Work out the finished part from the listing and answer in its coordinate system (mm). Round coordinates to 2 decimals unless told otherwise and drop trailing zeros. Loops run counter-clockwise (first coordinate to the right, second up) from the corner with the lowest first, then second, coordinate; pieces in that order, holes last. Notation, with made-up numbers: (-10, -32) -> (29, -32) arc R19 cw to (29, -18) -> close; hole circle Ø8 at (85.5, -18.75). An arc over 180 degrees is marked (long way). Write item = value, one per line. Start each with the question number.
```python
from build123d import *

# Parameters (mm, degrees)
SKETCH_W       = 190
SKETCH_H       = 82
SKETCH_R       = 1.65
PAD_DEPTH      = 0.75
PAD_DEPTH_BACK = 1.75
POCKET_DEPTH   = 5


with BuildPart() as part:
    # Sketch → Pad (new body, two sides)
    with BuildSketch(Plane.XZ) as pad_sk:
        Rectangle(SKETCH_W, SKETCH_H)
        with Locations((90, 30)):
            Circle(SKETCH_R, mode=Mode.SUBTRACT)
        with Locations((90, 10)):
            Circle(SKETCH_R, mode=Mode.SUBTRACT)
        with Locations((90, -30)):
            Circle(SKETCH_R, mode=Mode.SUBTRACT)
        with Locations((90, -10)):
            Circle(SKETCH_R, mode=Mode.SUBTRACT)
        with Locations((-90, 30)):
            Circle(SKETCH_R, mode=Mode.SUBTRACT)
        with Locations((-90, 10)):
            Circle(SKETCH_R, mode=Mode.SUBTRACT)
        with Locations((-90, -30)):
            Circle(SKETCH_R, mode=Mode.SUBTRACT)
        with Locations((-90, -10)):
            Circle(SKETCH_R, mode=Mode.SUBTRACT)
    extrude(amount=PAD_DEPTH)
    extrude(pad_sk.sketch, amount=-PAD_DEPTH_BACK)

    # Sketch001 → Pocket (cut)
    with BuildSketch(Plane.XZ.offset(0.75)):
        with BuildLine():
            Line((-80, -17), (-80, -33))
            ThreePointArc((-80, -33), (-79.414214, -34.414214), (-78, -35))
            Line((-78, -35), (-12, -35))
            ThreePointArc((-12, -35), (-10.585786, -34.414214), (-10, -33))
            Line((-10, -33), (-10, -17))
            ThreePointArc((-10, -17), (-10.585786, -15.585786), (-12, -15))
            Line((-12, -15), (-78, -15))
            ThreePointArc((-78, -15), (-79.414214, -15.585786), (-80, -17))
        make_face()
    extrude(amount=-POCKET_DEPTH, mode=Mode.SUBTRACT)


solid = part.part
```
Item 1: Section B-B (y = 0.85) is taken. Count the separate pieces of the cut face and the enclosed holes in it, then the cut area to 3 significant figures.
Item 2: Find the intervals of material crossed by line 1 along Z through (x, y) = (90, 0.8); line 2 along X through (y, z) = (0.8, -27); line 3 along Z through (x, y) = (-48, -0.55), in increasing order. Write a range as [from, to].
Item 3: Flat-ended cylindrical pins translate along their axes: pin 1 (3 mm diameter, centred on x = -90, z = 30, fed in from +Y); pin 2 (5.5 mm diameter, centred on x = 90, z = 30, fed in from -Y). Find the tip coordinate at first contact, or state that the pin passes through.
Item 4: Section A-A (x = -29) is taken. Determine the outline of the cut face in (y, z).
Worked answers:
q1.separate_pieces = 1
q1.enclosed_holes = 9
q1.area = 14,100 mm2
q2.line_1 = [-41, -31.65], [-28.35, -11.65], [-8.35, 8.35], [11.65, 28.35], [31.65, 41]
q2.line_2 = [-95, -80], [-10, 95]
q2.line_3 = [-41, -35], [-15, 41]
q3.pin_1 = through
q3.pin_2 = -0.75
q4.outline = (-0.75, -41) -> (1.75, -41) -> (1.75, -35) -> (-0.75, -35) -> close; (-0.75, -15) -> (1.75, -15) -> (1.75, 41) -> (-0.75, 41) -> close
